Can you work these out from the model? Positions are in its coordinate system, mm. Face numbers are marked on the shaded views. A direction names the side the tool comes from. Give positions to 0.01 mm unless a question says otherwise; leave off trailing zeros. Loops run counter-clockwise (first coordinate to the right, second up) from the corner with the lowest first, then second, coordinate; pieces in that order, holes last. Notation, with made-up numbers: M -10.5,44.5 L -0.5,44.5 A25 ccw -0.5,71.5 Z; hole C 65.5,55 d2. An arc over 180 degrees is marked long. Put each result on its own line as item: value. Start each with the question number.
1) Imagine slicing it at C-C (z = 26). Write out the boundary of the cut face in (x, y), then the cut area to 3 significant figures.
2) For the marked faces 1 and 2, which set-ups out of +Z, -Z, +X, -X, +Y, -Y let a thin tool reach every point of the face, with its end or its side?
3) Please list where these lines run through material, in increasing order: line 1 along Y through (x, z) = (61.5, -6.7) (3 decimals); line 2 along X through (y, z) = (24, 17); line 3 along Y through (x, z) = (36, -2.5). Write a range as from..to.
4) Imagine slicing it at B-B (y = 19). Write out the boundary of the cut face in (x, z), then the cut area to 3 significant figures.
5) Imagine slicing it at D-D (x = 82). Write out the boundary of the cut face in (y, z).
6) For P1, Ø1.9, axis at x = 61, y = 51, coming from the +Z side; P2, Ø1.5, axis at x = 67, y = 34.5, coming from the +Z side, each with a flat end and sliding along its axis, tell me the tip position at first contact or that it passes through.
7) If we mould it in two halves opening along Y, with no side actions, what happens to the marked faces 3, 4 and 5? For each: +Y half, -Y half, draft (parallel to the pull), parting line (faces both ways), or undercut.
8) Imagine slicing it at A-A (x = 3.5). Write out the boundary of the cut face in (y, z) (3 decimals), then the cut area to 3 significant figures.
from build123d import *

# Parameters (mm, degrees)
F0_W      = 100.33
F0_H      = 71.12
F0_W_2    = 90.17
F0_H_2    = 60.96
F1_DEPTH  = 5.08
F2_W      = 100.33
F2_H      = 71.12
F3_DEPTH  = 5.08
F0_R      = 1.375
F4_DEPTH  = 25.4
F5_R      = 3.1
F5_R_2    = 1.375
F6_DEPTH  = 3.556
F7_DEPTH  = 37.592
F8_W      = 13.716
F8_H      = 3.556
F9_DEPTH  = 5.08
F10_W     = 10.668
F10_H     = 5.715
F10_W_2   = 17.78
F10_H_2   = 9.144
F10_W_3   = 9.398
F10_H_3   = 8.89
F11_DEPTH = 5.08
F12_W     = 53.8226
F12_H     = 18.161
F13_DEPTH = 5.08
F14_R     = 1.905
F15_DEPTH = 71.121


with BuildPart() as f1:
    # F0 (on Top) → F1 (new body)
    with BuildSketch(Plane.XY):
        with Locations((42.545, 27.94)):
            Rectangle(F0_W, F0_H)
        with Locations((42.545, 27.94)):
            Rectangle(F0_W_2, F0_H_2, mode=Mode.SUBTRACT)
    extrude(amount=-F1_DEPTH)

    # F2 (on face) → F3 (join)
    with BuildSketch(Plane(origin=(0, 0, -5.08), x_dir=(1, 0, 0), z_dir=(0, 0, -1))):
        with Locations((42.545, -27.94)):
            Rectangle(F2_W, F2_H)
    extrude(amount=F3_DEPTH)

    # F0 (on Top) → F4 (cut)
    with BuildSketch(Plane.XY):
        with Locations((3.5, 52.38)):
            Circle(F0_R)
        with Locations((61.5, 52.38)):
            Circle(F0_R)
        with Locations((61.5, 3.5)):
            Circle(F0_R)
        with Locations((3.5, 3.5)):
            Circle(F0_R)
    extrude(amount=-F4_DEPTH, mode=Mode.SUBTRACT)

    # F5 (on face) → F6 (join)
    with BuildSketch(Plane.XY.offset(-5.08)):
        with Locations((3.5, 52.38)):
            Circle(F5_R)
        with Locations((3.5, 52.38)):
            Circle(F5_R_2, mode=Mode.SUBTRACT)
        with Locations((61.5, 52.38)):
            Circle(F5_R)
        with Locations((61.5, 52.38)):
            Circle(F5_R_2, mode=Mode.SUBTRACT)
        with Locations((61.5, 3.5)):
            Circle(F5_R)
        with Locations((61.5, 3.5)):
            Circle(F5_R_2, mode=Mode.SUBTRACT)
        with Locations((3.5, 3.5)):
            Circle(F5_R)
        with Locations((3.5, 3.5)):
            Circle(F5_R_2, mode=Mode.SUBTRACT)
    extrude(amount=F6_DEPTH)

    # F0 (on Top) → F7 (join)
    with BuildSketch(Plane.XY):
        with Locations((42.545, 27.94)):
            Rectangle(F0_W, F0_H)
        with Locations((42.545, 27.94)):
            Rectangle(F0_W_2, F0_H_2, mode=Mode.SUBTRACT)
    extrude(amount=F7_DEPTH)

    # F8 (on face) → F9 (cut, through all)
    with BuildSketch(Plane(origin=(-7.62, 0, 0), x_dir=(0, -1, 0), z_dir=(-1, 0, 0))):
        with Locations((-27.94, -2.032)):
            Rectangle(F8_W, F8_H)
    extrude(amount=-F9_DEPTH, mode=Mode.SUBTRACT)

    # F10 (on face) → F11 (cut, through all)
    with BuildSketch(Plane.XZ.offset(7.62)):
        with Locations((10.922, 1.5875)):
            Rectangle(F10_W, F10_H)
        with Locations((31.75, 3.302)):
            Rectangle(F10_W_2, F10_H_2)
        with Locations((53.594, 3.175)):
            Rectangle(F10_W_3, F10_H_3)
    extrude(amount=-F11_DEPTH, mode=Mode.SUBTRACT)

    # F12 (on face) → F13 (cut, through all)
    with BuildSketch(Plane.YZ.offset(92.71)):
        with Locations((28.8163, 7.8105)):
            Rectangle(F12_W, F12_H)
    extrude(amount=-F13_DEPTH, mode=Mode.SUBTRACT)

    # F14 (on face) → F15 (cut, through all)
    with BuildSketch(Plane.XZ.offset(7.62)):
        with Locations((31.9024, 19.304)):
            Circle(F14_R)
    extrude(amount=-F15_DEPTH, mode=Mode.SUBTRACT)


solid = f1.part
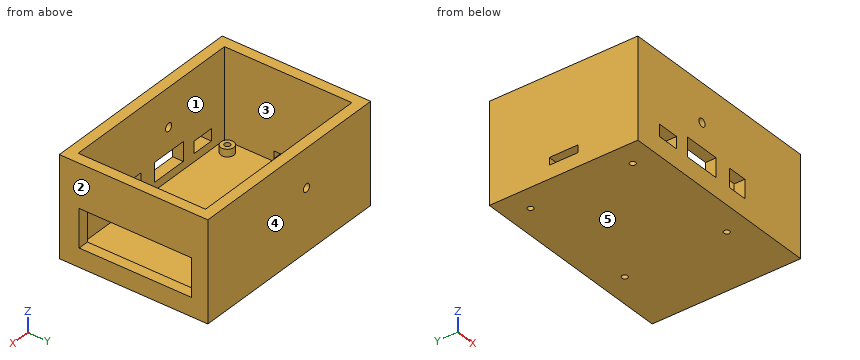
Recorded:
1. outline: M -7.62,-7.62 L 92.71,-7.62 L 92.71,63.5 L -7.62,63.5 Z; hole M -2.54,-2.54 L 87.63,-2.54 L 87.63,58.42 L -2.54,58.42 Z
1. area: 1,640 mm²
2. face 1: +Z
2. face 2: +Z, -Z, +X, +Y, -Y
3. line 1: -7.62..2.125, 4.875..51.005, 53.755..63.5
3. line 2: -7.62..-2.54, 87.63..92.71
3. line 3: -7.62..-2.54, 58.42..63.5
4. outline: M -7.62,-10.16 L 92.71,-10.16 L 92.71,-1.27 L 87.63,-1.27 L 87.63,-5.08 L -2.54,-5.08 L -2.54,37.59 L -7.62,37.59 Z; M 87.63,16.89 L 92.71,16.89 L 92.71,37.59 L 87.63,37.59 Z
4. area: 851 mm²
5. outline: M -7.62,-10.16 L 63.5,-10.16 L 63.5,37.59 L 58.42,37.59 L 58.42,-5.08 L -2.54,-5.08 L -2.54,37.59 L -7.62,37.59 Z
6. P1: z = -1.52
6. P2: z = -5.08
7. face 3: undercut
7. face 4: +Y half
7. face 5: draft
8. outline: M -7.62,-10.16 L 2.125,-10.16 L 2.125,-1.524 L 0.4,-1.524 L 0.4,-5.08 L -2.54,-5.08 L -2.54,37.592 L -7.62,37.592 Z; M 4.875,-10.16 L 51.005,-10.16 L 51.005,-1.524 L 49.28,-1.524 L 49.28,-5.08 L 6.6,-5.08 L 6.6,-1.524 L 4.875,-1.524 Z; M 53.755,-10.16 L 63.5,-10.16 L 63.5,37.592 L 58.42,37.592 L 58.42,-5.08 L 55.48,-5.08 L 55.48,-1.524 L 53.755,-1.524 Z
8. area: 791 mm²
